from build123d import *

# Parameters (mm, degrees)
F0_W     = 150
F0_H     = 150
F1_DEPTH = 25


with BuildPart() as f1:
    # F0 (on Top) → F1 (new body)
    with BuildSketch(Plane.XY):
        with Locations((-151.240738, 3.709819)):
            Rectangle(F0_W, F0_H)
        Polygon((-153.590513, 9.67208), (-147.252156, 8.725914), (-144.902381, 2.763653), (-148.890964, -2.252442), (-155.229321, -1.306276), (-157.579095, 4.655985), align=None, mode=Mode.SUBTRACT)
    extrude(amount=F1_DEPTH)


solid = f1.part
Build history of the part. All positions in model axes, mm. A direction names the side the tool comes from. Coordinates: 2 decimals unless noted, no trailing zeros. Use CSV: the item, a comma, the result in double quotes. Start each with the question number.
Q1. 3-axis set-ups, long thin cutter, end or side, ignore diameter. For faces 1 (the flat face through (-156.388, 1.633, 12.325)), 2 (the flat face through (-152, -71.29, 12)): which of +Z, -Z, +X, -X, +Y, -Y reach the whole face in a straight line?
Q2. Drill centre line: probe 1 along X at (y, z) = (5, 17.75). Where is it in solid material? Low to high.
Q3. Pull direction X, two halves, no side cores. Call faces 3 (the flat face through (-169, 5, 0)), 4 (the flat face through (-146.87, 0.29, 12.32)), 5 (the flat face through (-146.1, 5.8, 12.3)), 6 (the flat face through (-76.241, 3, 12)): released by +X, released by -X, zero draft, split by the parting line, or undercut.
Checked values:
1,face 1,"+Z, -Z"
1,face 2,"+Z, -Z, +X, -X, -Y"
2,probe 1,"x = -226.24 to -157.31, -145.78 to -76.24"
3,face 3,"zero draft"
3,face 4,"undercut"
3,face 5,"undercut"
3,face 6,"released by +X"
